Here's how the part is built. I have some questions about the finished solid (model axes, mm). Face numbers are marked on the shaded views. A direction names the side the tool comes from. Round coordinates to 2 decimals unless told otherwise and drop trailing zeros. Loops run counter-clockwise (first coordinate to the right, second up) from the corner with the lowest first, then second, coordinate; pieces in that order, holes last. Notation, with made-up numbers: M -30.75,-6.75 L 9.25,-6.75 A17 cw 9.25,25.25 Z; hole C 73,-36 d6. An arc over 180 degrees is marked long. Answer as a JSON object with one key per item and string values.
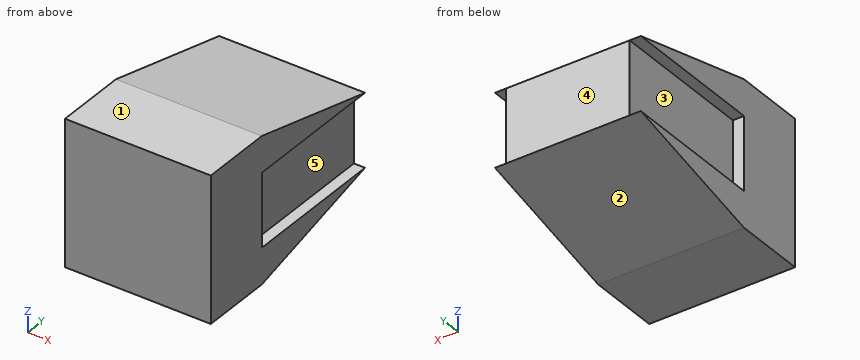
from build123d import *

# Parameters (mm, degrees)
F0_W     = 80.14
F0_H     = 79.66
F1_DEPTH = 39.53
F2_W     = 67.9
F2_H     = 40.24
F3_DEPTH = 80
F5_DEPTH = 80.14


with BuildPart() as f1:
    # F0 (on Front) → F1 (new body)
    with BuildSketch(Plane.XZ):
        Rectangle(F0_W, F0_H)
    extrude(amount=F1_DEPTH)

    # F2 (on face) → F3 (join)
    with BuildSketch(Plane(origin=(0, 0, 0), x_dir=(-1, 0, 0), z_dir=(0, 1, 0))):
        Rectangle(F2_W, F2_H)
    extrude(amount=F3_DEPTH)

    # F4 (on face) → F5 (join, through all)
    with BuildSketch(Plane.YZ.offset(40.07)):
        Polygon((80, 20.12), (0, 39.83), (0, 20.12), align=None)
        Polygon((80, -20.12), (0, -20.12), (0, -39.83), align=None)
        Polygon((0, 20.12), (0, 39.83), (-39.53, 39.83), (-39.53, -39.83), (0, -39.83), (0, -20.12), align=None)
    extrude(amount=-F5_DEPTH)


solid = f1.part
Item 1: I want a section at A-A, the plane z = -1. Please give me the cut outline in (x, y), then the cut area to 3 significant figures.
Resolved:
{"outline": "M -40.07,-39.53 L 40.07,-39.53 L 40.07,0 L 33.95,0 L 33.95,80 L -33.95,80 L -33.95,0 L -40.07,0 Z", "area": "8,600 mm²"}
Item 2: I want a section at B-B, the plane x = 12.5. Please give me the cut outline in (y, z), then the cut area to 3 significant figures.
Resolved:
{"outline": "M -39.53,-39.83 L 0,-39.83 L 80,-20.12 L 80,20.12 L 0,39.83 L -39.53,39.83 Z", "area": "7,940 mm²"}
Item 3: On a 3-axis mill with a long thin cutter (end or side, diameter ignored), from which of +Z, -Z, +X, -X, +Y, -Y can I reach the whole of each face in a straight line? I mean the marked faces 4 and 5. Say none if no direction works.
Resolved:
{"face 4": "+Z, -Z, +X, -X, +Y", "face 5": "+X, +Y"}
Item 4: I want a section at C-C, the plane y = 53.5. Please give me the cut outline in (x, z).
Resolved:
{"outline": "M -40.07,-26.65 L 40.07,-26.65 L 40.07,-20.12 L 33.95,-20.12 L 33.95,20.12 L 40.07,20.12 L 40.07,26.65 L -40.07,26.65 L -40.07,20.12 L -33.95,20.12 L -33.95,-20.12 L -40.07,-20.12 Z"}
Item 5: I want a section at D-D, the plane y = 2.5. Please give me the cut outline in (x, z), then the cut area to 3 significant figures.
Resolved:
{"outline": "M -40.07,-39.21 L 40.07,-39.21 L 40.07,-20.12 L 33.95,-20.12 L 33.95,20.12 L 40.07,20.12 L 40.07,39.21 L -40.07,39.21 L -40.07,20.12 L -33.95,20.12 L -33.95,-20.12 L -40.07,-20.12 Z", "area": "5,790 mm²"}
Item 6: I'm going to push flat-ended pins straight in: pin 1 Ø5 at (x, y) = (-23.5, 18) entering from +Z; pin 2 Ø3 at (x, y) = (-38.5, 25.5) entering from -Z; pin 3 Ø6.5 at (x, y) = (37, 49.5) entering from -Z. Where does each tip first touch, or does it pass through?
Resolved:
{"pin 1": "z = 36.01", "pin 2": "z = -33.92", "pin 3": "z = -28.44"}
Item 7: If we mould it in two halves opening along Z, with no side actions, what happens to the marked faces 1, 2 and 3? For each: pulls with the +Z half, pulls with the -Z half, needs draft (parallel to the pull), parting line crosses it, or undercut.
Resolved:
{"face 1": "pulls with the +Z half", "face 2": "pulls with the -Z half", "face 3": "undercut"}
Item 8: Please list where these lines run through material, in increasing order: probe 1 along X at (y, z) = (63, -8); probe 2 along Z at (x, y) = (34, 27); probe 3 along Z at (x, y) = (25.5, 61.5). Write a range as from..to.
Resolved:
{"probe 1": "-33.95..33.95", "probe 2": "-33.18..-20.12, 20.12..33.18", "probe 3": "-24.68..24.68"}
